Geometry: final body of the model. Coordinates: model frame, mm. Face numbers are marked on the shaded views. Coordinates: 2 decimals unless noted, no trailing zeros. Loops run counter-clockwise (first coordinate to the right, second up) from the corner with the lowest first, then second, coordinate; pieces in that order, holes last. Notation, with made-up numbers: (13, -33.75) - (39, -33.75) arc R35 ccw to (39, 3.25) - close; hole circle Ø6 at (59, 38). An arc over 180 degrees is marked (long way). Return JSON: item names as keys, results as strings.
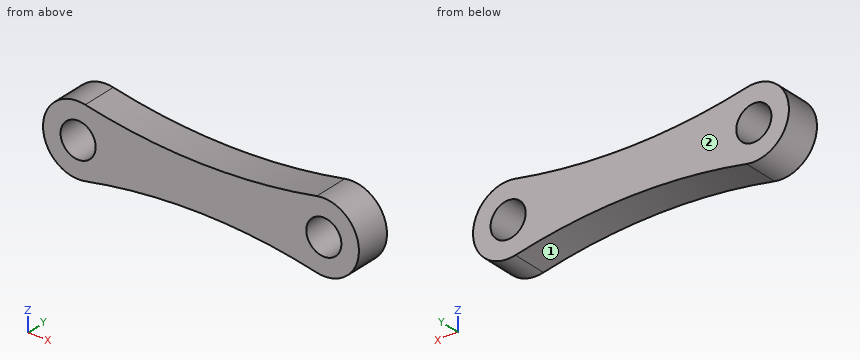
Autodesk Inventor part; units mm, degrees
ref_plane "YZ Plane" through (0, 0, 0) normal (1, 0, 0) x (0, 1, 0)
ref_plane "XZ Plane" through (0, 0, 0) normal (0, 1, 0) x (-1, 0, 0)
ref_plane "XY Plane" through (0, 0, 0) normal (0, 0, 1) x (1, 0, 0)
sketch "Sketch1" plane through (0, 0, 0) normal (0, 1, 0) x (-1, 0, 0)
  line L0 (-15.1311, 4.4797) -> (19.8689, 4.4797)
  circle A0 centre (19.8689, 4.4797) radius 2.5
  circle A1 centre (-15.1311, 4.4797) radius 2.5
  circle A2 centre (-15.1311, 4.4797) radius 5
  circle A3 centre (19.8689, 4.4797) radius 5
  line L1 (2.3689, 4.4797) -> (2.3689, 1.3284)
  line L2 (2.3689, 1.3284) -> (2.3689, 4.4797)
  line L3 (2.3689, 4.4797) -> (2.3689, 7.6857)
  arc A4 (-14.1166, 9.3757) -> (18.8544, 9.3757) centre (2.3689, 88.9357) ccw
  arc A5 (18.8242, -0.4099) -> (-14.0864, -0.4099) centre (2.3689, -77.427) ccw
  point P0 (0, 0)
  point P1 (7.7903, 4.509)
  dimension "d0" = 35
  dimension "d1" = 5
  dimension "d2" = 5
  dimension "d3" = 10
  dimension "d4" = 10
extrude "Extrusion1" add sketch "Sketch1" along normal blind 5
properties part number "body-tail"
Item 1: Section query B-B, the plane z = 5. Return loops of the section in (x, y).
Worked out:
{"outline": "(-24.84, 0) - (-22.31, 0) - (-22.31, 5) - (-24.84, 5) - close; (-17.42, 0) - (12.69, 0) - (12.69, 5) - (-17.42, 5) - close; (17.58, 0) - (20.1, 0) - (20.1, 5) - (17.58, 5) - close"}
Item 2: Mould query, pull axis X, two halves, no side actions, for the marked faces 1 and 2. Classes: +X half, -X half, draft (parallel to the pull), parting line (faces both ways), or undercut.
Worked out:
{"face 1": "undercut", "face 2": "draft"}
Item 3: Section query A-A, the plane x = 15.5. Return loops of the section in (y, z), and give its area (3 significant figures).
Worked out:
{"outline": "(0, -0.51) - (5, -0.51) - (5, 2.01) - (0, 2.01) - close; (0, 6.95) - (5, 6.95) - (5, 9.47) - (0, 9.47) - close", "area": "25.1 mm^2"}
Item 4: Ray query, probe 1 along Z at (x, y) = (-20, 1.95); probe 2 along X at (y, z) = (3.4, 2.25); probe 3 along X at (y, z) = (3.15, 6.5). Return the intervals inside material, ascending. Write a range as from..to.
Worked out:
{"probe 1": "-0.52..1.98, 6.98..9.48", "probe 2": "-24.34..-21, -18.74..14, 16.26..19.61", "probe 3": "-24.44..-21.34, -18.4..13.66, 16.6..19.7"}
Item 5: First-contact query: pin 1 Ø3 at (x, y) = (13.5, 1) entering from -Z; pin 2 Ø2 at (x, y) = (-4, 1) entering from -Z; pin 3 Ø5 at (x, z) = (-1, 4) entering from -Y. Flat tips, straight axial feed; report the tip coordinate or a pass-through.
Worked out:
{"pin 1": "z = -0.52", "pin 2": "z = 1.28", "pin 3": "y = 0"}
Item 6: Section query D-D, the plane y = 2.5. Return loops of the section in (x, z), and give its area (3 significant figures).
Worked out:
{"outline": "(-18.85, 9.38) arc R5 ccw (long way) to (-18.82, -0.41) arc R78.76 cw to (14.09, -0.41) arc R5 ccw (long way) to (14.12, 9.38) arc R81.25 cw to start; hole circle Ø5 at (-19.87, 4.48); hole circle Ø5 at (15.13, 4.48)", "area": "307 mm^2"}
